from build123d import *

# Parameters (mm, degrees)
SCHIZZO1_R                   = 16.05
ESTRUSIONE_ESTRUSIONE1_DEPTH = 3.8
SCHIZZO2_R                   = 13.4
ESTRUSIONE_ESTRUSIONE2_DEPTH = 3
SMUSSO1_SIZE                 = 2.65
RACCORDO1_R                  = 1
SCHIZZO3_R                   = 13.25
TAGLIO_ESTRUSIONE1_DEPTH     = 5
SMUSSO2_SIZE                 = 1.5


with BuildPart() as part:
    # Schizzo1 → Estrusione-Estrusione1 (new body)
    with BuildSketch(Plane.XY):
        with Locations(Location((0, 0, 0), (0, 0, 180))):
            Circle(SCHIZZO1_R)
    extrude(amount=ESTRUSIONE_ESTRUSIONE1_DEPTH)

    # Schizzo2 → Estrusione-Estrusione2 (add)
    with BuildSketch(Plane.XY.offset(3.8)):
        Circle(SCHIZZO2_R)
    extrude(amount=ESTRUSIONE_ESTRUSIONE2_DEPTH)

    # Smusso1
    smusso1_edges = [part.edges().sort_by_distance(p)[0] for p in [
        (16.05, 0, 3.8),
    ]]
    chamfer(smusso1_edges, length=SMUSSO1_SIZE - 0.0001)  # a hair under: the kernel refuses the full size

    # Raccordo1
    raccordo1_edges = [part.edges().sort_by_distance(p)[0] for p in [
        (-13.4, 0, 6.8),
    ]]
    fillet(raccordo1_edges, radius=RACCORDO1_R)

    # Schizzo3 → Taglio-Estrusione1 (cut)
    with BuildSketch(Plane(origin=(0, 0, 0), x_dir=(-1, 0, 0), z_dir=(0, 0, -1))):
        Circle(SCHIZZO3_R)
    extrude(amount=-TAGLIO_ESTRUSIONE1_DEPTH, mode=Mode.SUBTRACT)

    # Smusso2
    smusso2_edges = [part.edges().sort_by_distance(p)[0] for p in [
        (13.25, 0, 0),
    ]]
    chamfer(smusso2_edges, length=SMUSSO2_SIZE)


solid = part.part
The model under review builds one solid part; all positions refer to its coordinate system, in mm. A direction names the side the tool comes from. Round coordinates to 2 decimals unless told otherwise and drop trailing zeros. Order: outer loops, then holes, each group sorted by start corner. A loop starts at its lowest first (then second) coordinate and runs counter-clockwise, first axis right, second up. Notation, with made-up numbers: (-18.5, 8) -> (31.5, 8) arc R27 cw to (31.5, 30) -> close; hole circle Ø5 at (39, -13). An arc over 180 degrees is marked (long way). Return JSON: item names as keys, results as strings.
1. Take a section at D-D (z = 6.25). Write out the cut boundary in (x, y), then the cut area to 3 significant figures.
Answer block:
{"outline": "circle Ø26.59 at (0, 0)", "area": "555 mm²"}
2. For L1, parallel to Y at x = 0, z = 3.35; L2, parallel to Y at x = -2, z = 4; L3, parallel to Z at x = 4.5, y = 4, list the stretches that pass through material, from the lowest coordinate up. Write a range as [from, to].
Answer block:
{"L1": "y = [-13.85, -13.25], [13.25, 13.85]", "L2": "y = [-13.25, -13.1], [13.1, 13.25]", "L3": "z = [5, 6.8]"}
3. For faces 1 (the face through (-10.6, -8.2, 4.8)), 2 (the face through (0, 0, 6.8)), list the 3-axis set-ups (+Z, -Z, +X, -X, +Y, -Y) from which the entire face can be reached by the end or side of a thin tool; tool diameter is ignored.
Answer block:
{"face 1": "+Z", "face 2": "+Z, +X, -X, +Y, -Y"}
4. Insertion check: P1, Ø1.5, axis at x = 6.5, z = 2.5, coming from the -Y side; P2, Ø8, axis at x = -6.5, y = 6, coming from the -Z side; P3, Ø4, axis at x = -11, z = 1.5, coming from the +Y side. Each pin has a flat end and moves straight along its axis. Give the tip position at first contact, or say it passes through.
Answer block:
{"P1": "stops at y = -14.08", "P2": "stops at z = 5", "P3": "stops at y = 13.27"}
5. The part is to be moulded in two halves that separate along X. For faces 3 (the face through (-14.2, 4.7, 0)), 4 (the face through (0, 0, 5)), 5 (the face through (-7.123, 11.172, 3.226)), 6 (the face through (-15.31, -4.82, 0.57)), say which applies: +X half, -X half, draft (parallel to the pull), parting line (faces both ways), or undercut.
Answer block:
{"face 3": "draft", "face 4": "undercut", "face 5": "undercut", "face 6": "parting line"}
6. Take a section at C-C (z = 3). Write out the cut boundary in (x, y), then the cut area to 3 significant figures.
Answer block:
{"outline": "circle Ø28.4 at (0, 0); hole circle Ø26.5 at (0, 0)", "area": "81.9 mm²"}
